from build123d import *

# Parameters (mm, degrees)
F0_W     = 1524
F0_H     = 1524
F0_W_2   = 1473.2
F0_H_2   = 1473.2
F1_DEPTH = 25.4
F2_W     = 25.4
F2_H     = 1473.2
F2_H_2   = 1468.964992
F2_H_3   = 1466.467655
F2_H_4   = 1472.886331
F3_DEPTH = 25.4
F4_W     = 1471.939683
F4_H     = 25.4
F4_W_2   = 1503.417969
F5_DEPTH = 25.4


with BuildPart() as f1:
    # F0 (on Front) → F1 (new body)
    with BuildSketch(Plane.XZ):
        with Locations((-33.591984, 108.689165)):
            Rectangle(F0_W, F0_H)
        with Locations((-33.591984, 108.689165)):
            Rectangle(F0_W_2, F0_H_2, mode=Mode.SUBTRACT)
    extrude(amount=F1_DEPTH)

    # F2 (on Front) → F3 (join)
    with BuildSketch(Plane.XZ):
        with Locations((-583.836417, 104.738611)):
            Rectangle(F2_W, F2_H)
        Polygon((-367.961303, 851.760401), (-393.361303, 838.36392), (-393.361303, -634.83608), (-367.961303, -621.439599), align=None)
        Polygon((-190.161303, -634.83608), (-190.161303, 838.36392), (-215.561303, 838.36392), (-215.561303, -621.439599), align=None)
        with Locations((0.338697, 103.881424)):
            Rectangle(F2_W, F2_H_2)
        with Locations((203.52335, 102.632756)):
            Rectangle(F2_W, F2_H_3)
        Polygon((419.42335, -612.278187), (419.42335, 835.866583), (394.02335, 860.921813), (394.02335, -612.278187), align=None)
        with Locations((609.536889, 111.949723)):
            Rectangle(F2_W, F2_H_4)
    extrude(amount=F3_DEPTH)

    # F4 (on Front) → F5 (join)
    with BuildSketch(Plane.XZ):
        with Locations((-34.39182, 223.449667)):
            Rectangle(F4_W, F4_H)
        with Locations((-34.39182, -201.515604)):
            Rectangle(F4_W, F4_H)
        with Locations((-18.652677, 586.853881)):
            Rectangle(F4_W_2, F4_H)
    extrude(amount=F5_DEPTH)


solid = f1.part
Input: part model. Units: mm. Frame: model coordinates. Give positions to 0.01 mm unless a question says otherwise; leave off trailing zeros. Loops run counter-clockwise (first coordinate to the right, second up) from the corner with the lowest first, then second, coordinate; pieces in that order, holes last. Notation, with made-up numbers: (-22, 23.5) - (12, 23.5) arc R13 cw to (12, 40.5) - close; hole circle Ø10 at (23, 29). An arc over 180 degrees is marked (long way). Use CSV: the item, a comma, the result in double quotes. Start each with the question number.
Item 1: Section B-B on z = 180.5. State how many separate pieces and enclosed holes the cut face has, then the cut area to 3 significant figures.
Item 2: Section A-A on x = 266. Return loops of the section in (y, z), then the cut area to 3 significant figures.
Item 3: Contact query for a flat-ended pin moving along its axis: P1, Ø12, axis at y = -17, z = 303, coming from the +X side. Output: stop coordinate, or through.
Item 4: Line query: line 1 (Z direction, x = -556, y = -12.75); line 2 (Z direction, x = -586, y = -6.5); line 3 (X direction, y = -11.75, z = 212.5). Output: solid intervals per line, ascending.
Ans:
1,separate pieces,"9"
1,enclosed holes,"0"
1,area,"5,810 mm2"
2,outline,"(-25.4, -653.31) - (0, -653.31) - (0, -627.91) - (-25.4, -627.91) - close; (-25.4, -214.22) - (0, -214.22) - (0, -188.82) - (-25.4, -188.82) - close; (-25.4, 210.75) - (0, 210.75) - (0, 236.15) - (-25.4, 236.15) - close; (-25.4, 574.15) - (0, 574.15) - (0, 599.55) - (-25.4, 599.55) - close; (-25.4, 845.29) - (0, 845.29) - (0, 870.69) - (-25.4, 870.69) - close"
2,area,"3,230 mm2"
3,P1,"stops at x = 728.41"
4,line 1,"z = -653.31 to -627.91, -214.22 to -188.82, 210.75 to 236.15, 574.15 to 599.55, 845.29 to 870.69"
4,line 2,"z = -653.31 to 841.34, 845.29 to 870.69"
4,line 3,"x = -795.59 to 701.58, 703.01 to 728.41"
